from build123d import *

# Parameters (mm, degrees)
SKETCH1_R           = 3.2
SKETCH1_R_2         = 14
BOSS_EXTRUDE1_DEPTH = 6.35


with BuildPart() as part:
    # Sketch1 → Boss-Extrude1 (new body)
    with BuildSketch(Plane.XY):
        Polygon((-647.460250444, -317.619540534), (-477.475995614, -23.198174681), (-442.475995614, -23.198174681), (-272.491740783, -317.619540534), (-289.991740783, -347.930429667), (-629.960250444, -347.930429667), align=None)
        with Locations((-581.209182953, -222.869325584)):
            Circle(SKETCH1_R, mode=Mode.SUBTRACT)
        with Locations((-528.649182953, -131.832735139)):
            Circle(SKETCH1_R, mode=Mode.SUBTRACT)
        with Locations((-500.577727615, -148.011529753)):
            Circle(SKETCH1_R, mode=Mode.SUBTRACT)
        with Locations((-553.136815613, -239.046537702)):
            Circle(SKETCH1_R, mode=Mode.SUBTRACT)
        with Locations((-367.294158494, -238.209054553)):
            Circle(SKETCH1_R, mode=Mode.SUBTRACT)
        with Locations((-419.854158494, -147.172464107)):
            Circle(SKETCH1_R, mode=Mode.SUBTRACT)
        with Locations((-391.545684719, -131.412060795)):
            Circle(SKETCH1_R, mode=Mode.SUBTRACT)
        with Locations((-338.985684719, -222.448651241)):
            Circle(SKETCH1_R, mode=Mode.SUBTRACT)
        with Locations((-511.800751787, -305.530429667)):
            Circle(SKETCH1_R, mode=Mode.SUBTRACT)
        with Locations((-406.680508256, -305.530429667)):
            Circle(SKETCH1_R, mode=Mode.SUBTRACT)
        with Locations((-406.680630022, -337.930429667)):
            Circle(SKETCH1_R, mode=Mode.SUBTRACT)
        with Locations((-511.800630022, -337.930429667)):
            Circle(SKETCH1_R, mode=Mode.SUBTRACT)
        with Locations((-459.807870528, -114.054080446)):
            Circle(SKETCH1_R_2, mode=Mode.SUBTRACT)
        with Locations((-358.022290508, -290.351876517)):
            Circle(SKETCH1_R_2, mode=Mode.SUBTRACT)
        with Locations((-561.593450547, -290.351876517)):
            Circle(SKETCH1_R_2, mode=Mode.SUBTRACT)
    extrude(amount=-BOSS_EXTRUDE1_DEPTH)


solid = part.part
Work out the finished part from the listing and answer in its coordinate system (mm). Coordinates: 2 decimals unless noted, no trailing zeros. Loops run counter-clockwise (first coordinate to the right, second up) from the corner with the lowest first, then second, coordinate; pieces in that order, holes last. Notation, with made-up numbers: M 76.5,-17.5 L 98.5,-17.5 A23 ccw 98.5,-9.5 Z; hole C 46.5,25.5 d10. An arc over 180 degrees is marked long. Answer in a Markdown table with one row per item. Add a question column.
1. Find section D-D, the plane x = -328.5. Write down the section's boundary in (y, z).
2. Find section C-C, the plane x = -566.5. Write down the section's boundary in (y, z).
3. Flat-ended cylindrical pins translate along their axes: P1, Ø4, axis at x = -338.99, y = -222.45, coming from the -Z side; P2, Ø1, axis at y = -100, z = -2.5, coming from the +X side; P3, Ø3, axis at x = -422.5, z = -3, coming from the +Y side. Find the tip coordinate at first contact, or state that the pin passes through.
4. Find section A-A, the plane y = -298. Write down the section's boundary in (x, z).
5. Consider L1, parallel to Y at x = -367, z = -0.5; L2, parallel to X at y = -283.5, z = -3; L3, parallel to X at y = -222, z = -5.25. Determine where each line is inside the solid, lowest interval first.
6. The mould has two halves that part along Y. Classify faces 1 (the flat face through (-563.66, -172.47, -3.13)), 2 (the flat face through (-457, -219, -6.35)), 3 (the flat face through (-281.119, -332.563, -3.131)), 4 (the cylindrical face through (-446.875, -119.416, -3.131)): pulls with the +Y half, pulls with the -Y half, needs draft (parallel to the pull), parting line crosses it, or undercut.
7. Find section B-B, the plane z = -4. State how many separate pieces and enclosed holes the cut face has, then the cut area to 3 significant figures.
Reported:
| question | item | result |
|---|---|---|
| 1 | outline | M -347.93,-6.35 L -220.61,-6.35 L -220.61,0 L -347.93,0 Z |
| 2 | outline | M -347.93,-6.35 L -303.46,-6.35 L -303.46,0 L -347.93,0 Z; M -277.24,-6.35 L -177.39,-6.35 L -177.39,0 L -277.24,0 Z |
| 3 | P1 | passes through |
| 3 | P2 | stops at x = -397.85 |
| 3 | P3 | stops at y = -55.2 |
| 4 | outline | M -636.13,-6.35 L -573.32,-6.35 L -573.32,0 L -636.13,0 Z; M -549.87,-6.35 L -369.75,-6.35 L -369.75,0 L -549.87,0 Z; M -346.3,-6.35 L -283.82,-6.35 L -283.82,0 L -346.3,0 Z |
| 5 | L1 | y = -347.93 to -301.09, -279.61 to -241.4, -235.02 to -153.93 |
| 5 | L2 | x = -627.76 to -573.8, -549.38 to -370.23, -345.81 to -292.19 |
| 5 | L3 | x = -592.25 to -584.29, -578.13 to -342.15, -335.82 to -327.7 |
| 6 | face 1 | pulls with the +Y half |
| 6 | face 2 | needs draft |
| 6 | face 3 | pulls with the -Y half |
| 6 | face 4 | undercut |
| 7 | separate pieces | 1 |
| 7 | enclosed holes | 15 |
| 7 | area | 69,000 mm^2 |
